Geometry: final body of the model. Coordinates: model frame, mm. A direction names the side the tool comes from. Round coordinates to 2 decimals unless told otherwise and drop trailing zeros. Order: outer loops, then holes, each group sorted by start corner. A loop starts at its lowest first (then second) coordinate and runs counter-clockwise, first axis right, second up. Notation, with made-up numbers: (40, -33) -> (73, -33) arc R34 cw to (73, 1) -> close; hole circle Ø9 at (82, 68). An arc over 180 degrees is marked (long way). Put each result on its own line as item: value.
```python
from build123d import *

# Parameters (mm, degrees)
SKETCH_1_W          = 265
SKETCH_1_H          = 40
EXTRUDE_1_DEPTH     = 1.5
SKETCH_2_R          = 11
SKETCH_2_R_2        = 2.1
CUT_EXTRUDE_1_DEPTH = 135.009328034
SKETCH_3_R          = 2.1
SKETCH_3_R_2        = 11
SKETCH_3_R_3        = 1.7
CUT_EXTRUDE_2_DEPTH = 135.009328034
SKETCH_4_R          = 1.7
CUT_EXTRUDE_3_DEPTH = 135.009328034


with BuildPart() as part:
    # 草图1 → 凸台-拉伸1 (new body)
    with BuildSketch(Plane.XY):
        Rectangle(SKETCH_1_W, SKETCH_1_H)
    extrude(amount=EXTRUDE_1_DEPTH)

    # 草图2 → 切除-拉伸1 (cut, through all)
    with BuildSketch(Plane.XY.offset(1.5)):
        with Locations((85, 0)):
            Circle(SKETCH_2_R)
        with Locations((55, 0)):
            Circle(SKETCH_2_R)
        with Locations((0, -15)):
            Circle(SKETCH_2_R_2)
        with Locations((30, 15)):
            Circle(SKETCH_2_R_2)
        with Locations((-30, 15)):
            Circle(SKETCH_2_R_2)
        with Locations((-55, 0)):
            Circle(SKETCH_2_R)
        with Locations((-85, 0)):
            Circle(SKETCH_2_R)
        with BuildLine():
            Line((30, -8.5), (30, 5.394448725))
            ThreePointArc((30, 5.394448725), (29.207786888, 6.716960623), (27.667949706, 6.642524166))
            Line((27.667949706, 6.642524166), (6.826276619, -7.251924558))
            ThreePointArc((6.826276619, -7.251924558), (6.222688873, -8.934676223), (7.658326913, -10))
            Line((7.658326913, -10), (28.5, -10))
            ThreePointArc((28.5, -10), (29.560660172, -9.560660172), (30, -8.5))
        make_face()
        with BuildLine():
            Line((3.832050294, -5.642524166), (23.173723381, 7.251924558))
            ThreePointArc((23.173723381, 7.251924558), (23.777311127, 8.934676223), (22.341673087, 10))
            Line((22.341673087, 10), (3, 10))
            ThreePointArc((3, 10), (1.939339828, 9.560660172), (1.5, 8.5))
            Line((1.5, 8.5), (1.5, -4.394448725))
            ThreePointArc((1.5, -4.394448725), (2.292213112, -5.716960623), (3.832050294, -5.642524166))
        make_face()
        with BuildLine():
            Line((-1.5, -4.394448725), (-1.5, 8.5))
            ThreePointArc((-1.5, 8.5), (-1.939339828, 9.560660172), (-3, 10))
            Line((-3, 10), (-22.341673087, 10))
            ThreePointArc((-22.341673087, 10), (-23.777311127, 8.934676223), (-23.173723381, 7.251924558))
            Line((-23.173723381, 7.251924558), (-3.832050294, -5.642524166))
            ThreePointArc((-3.832050294, -5.642524166), (-2.292213112, -5.716960623), (-1.5, -4.394448725))
        make_face()
        with BuildLine():
            Line((-6.826276619, -7.251924558), (-27.667949706, 6.642524166))
            ThreePointArc((-27.667949706, 6.642524166), (-29.207786888, 6.716960623), (-30, 5.394448725))
            Line((-30, 5.394448725), (-30, -8.5))
            ThreePointArc((-30, -8.5), (-29.560660172, -9.560660172), (-28.5, -10))
            Line((-28.5, -10), (-7.658326913, -10))
            ThreePointArc((-7.658326913, -10), (-6.222688873, -8.934676223), (-6.826276619, -7.251924558))
        make_face()
    extrude(amount=-CUT_EXTRUDE_1_DEPTH, mode=Mode.SUBTRACT)

    # 草图3 → 切除-拉伸2 (cut, through all)
    with BuildSketch(Plane(origin=(0, 0, 0), x_dir=(-1, 0, 0), z_dir=(0, 0, -1))):
        with Locations(Location((0, -15, 0), (0, 0, 180))):
            Circle(SKETCH_3_R)
        with Locations(Location((-30, 15, 0), (0, 0, 180))):
            Circle(SKETCH_3_R)
        with Locations(Location((30, 15, 0), (0, 0, 180))):
            Circle(SKETCH_3_R)
        with Locations(Location((85, 0, 0), (0, 0, 180))):
            Circle(SKETCH_3_R_2)
        with Locations(Location((55, 0, 0), (0, 0, 180))):
            Circle(SKETCH_3_R_2)
        with Locations(Location((-55, 0, 0), (0, 0, 180))):
            Circle(SKETCH_3_R_2)
        with Locations(Location((-85, 0, 0), (0, 0, 180))):
            Circle(SKETCH_3_R_2)
        with Locations((-55, -15)):
            Circle(SKETCH_3_R_3)
        with Locations((55, 15)):
            Circle(SKETCH_3_R_3)
        with Locations((-70, 0)):
            Circle(SKETCH_3_R_3)
        with Locations((-55, 15)):
            Circle(SKETCH_3_R_3)
        with Locations((85, 15)):
            Circle(SKETCH_3_R_3)
        with Locations((-85, 15)):
            Circle(SKETCH_3_R_3)
        with Locations((55, -15)):
            Circle(SKETCH_3_R_3)
        with Locations((85, -15)):
            Circle(SKETCH_3_R_3)
        with Locations((-37, 0)):
            Circle(SKETCH_3_R_3)
        with Locations((37, 0)):
            Circle(SKETCH_3_R_3)
        with Locations((109.5, 0)):
            Circle(SKETCH_3_R_3)
        with Locations((-85, -15)):
            Circle(SKETCH_3_R_3)
        with Locations((-109.5, 0)):
            Circle(SKETCH_3_R_3)
        with Locations((70, 0)):
            Circle(SKETCH_3_R_3)
        with BuildLine():
            Line((-1.5, -4.394448725), (-1.5, 8.5))
            ThreePointArc((-1.5, 8.5), (-1.939339828, 9.560660172), (-3, 10))
            Line((-3, 10), (-22.341673087, 10))
            ThreePointArc((-22.341673087, 10), (-23.777311127, 8.934676223), (-23.173723381, 7.251924558))
            Line((-23.173723381, 7.251924558), (-3.832050294, -5.642524166))
            ThreePointArc((-3.832050294, -5.642524166), (-2.292213112, -5.716960623), (-1.5, -4.394448725))
        make_face()
        with BuildLine():
            Line((30, -8.5), (30, 5.394448725))
            ThreePointArc((30, 5.394448725), (29.207786888, 6.716960623), (27.667949706, 6.642524166))
            Line((27.667949706, 6.642524166), (6.826276619, -7.251924558))
            ThreePointArc((6.826276619, -7.251924558), (6.222688873, -8.934676223), (7.658326913, -10))
            Line((7.658326913, -10), (28.5, -10))
            ThreePointArc((28.5, -10), (29.560660172, -9.560660172), (30, -8.5))
        make_face()
        with BuildLine():
            Line((3.832050294, -5.642524166), (23.173723381, 7.251924558))
            ThreePointArc((23.173723381, 7.251924558), (23.777311127, 8.934676223), (22.341673087, 10))
            Line((22.341673087, 10), (3, 10))
            ThreePointArc((3, 10), (1.939339828, 9.560660172), (1.5, 8.5))
            Line((1.5, 8.5), (1.5, -4.394448725))
            ThreePointArc((1.5, -4.394448725), (2.292213112, -5.716960623), (3.832050294, -5.642524166))
        make_face()
        with BuildLine():
            Line((-6.826276619, -7.251924558), (-27.667949706, 6.642524166))
            ThreePointArc((-27.667949706, 6.642524166), (-29.207786888, 6.716960623), (-30, 5.394448725))
            Line((-30, 5.394448725), (-30, -8.5))
            ThreePointArc((-30, -8.5), (-29.560660172, -9.560660172), (-28.5, -10))
            Line((-28.5, -10), (-7.658326913, -10))
            ThreePointArc((-7.658326913, -10), (-6.222688873, -8.934676223), (-6.826276619, -7.251924558))
        make_face()
    extrude(amount=-CUT_EXTRUDE_2_DEPTH, mode=Mode.SUBTRACT)

    # 草图4 → 切除-拉伸3 (cut, through all)
    with BuildSketch(Plane(origin=(0, 0, 0), x_dir=(-1, 0, 0), z_dir=(0, 0, -1))):
        with Locations((-129, -16)):
            Circle(SKETCH_4_R)
        with Locations((-129, 16)):
            Circle(SKETCH_4_R)
        with Locations((-117, -16)):
            Circle(SKETCH_4_R)
        with Locations((-117, 16)):
            Circle(SKETCH_4_R)
        with Locations(Location((117, 16, 0), (0, 0, 180))):
            Circle(SKETCH_4_R)
        with Locations(Location((117, -16, 0), (0, 0, 180))):
            Circle(SKETCH_4_R)
        with Locations(Location((129, 16, 0), (0, 0, 180))):
            Circle(SKETCH_4_R)
        with Locations(Location((129, -16, 0), (0, 0, 180))):
            Circle(SKETCH_4_R)
    extrude(amount=-CUT_EXTRUDE_3_DEPTH, mode=Mode.SUBTRACT)


solid = part.part
```
1. Contact query for flat-ended pins moving along their axis: P1, Ø3, axis at x = -85, y = 15, coming from the -Z side; P2, Ø4.5, axis at x = -117, y = -16, coming from the +Z side. Output: stop coordinate, or through.
Ans:
P1: through
P2: z = 1.5
2. Set-up query: faces 1 (the face through (-2, -9, 0)), 2 (the face through (13.367, 0.714, 0.76)). Return all of +Z, -Z, +X, -X, +Y, -Y with unobstructed straight access to the full face (end or side cutting, diameter ignored); none if empty.
Ans:
face 1: -Z, +X, -X, +Y, -Y
face 2: +Z, -Z
3. Cut plane B-B on z = 0.9. State how many separate pieces and enclosed holes the cut face has, and give its area (3 significant figures).
Ans:
separate pieces: 1
enclosed holes: 33
area: 7,930 mm²
4. Draft query along X for faces 3 (the face through (44, 0, 1)), 4 (the face through (-2, -9, 1.5)). Return one class per face: +X half, -X half, draft (parallel to the pull), parting line (faces both ways), or undercut.
Ans:
face 3: undercut
face 4: draft
5. Material intervals for probe 1 along Y at (x, z) = (117, 0.55); probe 2 along Y at (x, z) = (85, 0.4); probe 3 along X at (y, z) = (-17.5, 0.75), sorted ascending.
Ans:
probe 1: -20 to -17.7, -14.3 to 14.3, 17.7 to 20
probe 2: -20 to -16.7, -13.3 to -11, 11 to 13.3, 16.7 to 20
probe 3: -132.5 to -129.8, -128.2 to -117.8, -116.2 to 116.2, 117.8 to 128.2, 129.8 to 132.5
6. Cut plane A-A on x = 48. Return loops of the section in (y, z).
Ans:
outline: (-20, 0) -> (-8.49, 0) -> (-8.49, 1.5) -> (-20, 1.5) -> close; (8.49, 0) -> (20, 0) -> (20, 1.5) -> (8.49, 1.5) -> close
